from build123d import *

# Parameters (mm, degrees)
F0_R     = 140
F0_R_2   = 12.7
F0_R_3   = 87.5
F1_DEPTH = 15


with BuildPart() as f1:
    # F0 (on Front) → F1 (new body)
    with BuildSketch(Plane.XZ):
        Circle(F0_R)
        with Locations((-82.943625, -82.943625)):
            Circle(F0_R_2, mode=Mode.SUBTRACT)
        with Locations((0, -117.3)):
            Circle(F0_R_2, mode=Mode.SUBTRACT)
        with Locations((82.943625, -82.943625)):
            Circle(F0_R_2, mode=Mode.SUBTRACT)
        with Locations((-117.3, 0)):
            Circle(F0_R_2, mode=Mode.SUBTRACT)
        with Locations((-82.943625, 82.943625)):
            Circle(F0_R_2, mode=Mode.SUBTRACT)
        Circle(F0_R_3, mode=Mode.SUBTRACT)
        with Locations((117.3, 0)):
            Circle(F0_R_2, mode=Mode.SUBTRACT)
        with Locations((0, 117.3)):
            Circle(F0_R_2, mode=Mode.SUBTRACT)
        with Locations((82.943625, 82.943625)):
            Circle(F0_R_2, mode=Mode.SUBTRACT)
    extrude(amount=F1_DEPTH)


solid = f1.part
Part model, mm, in its own coordinate system. Give positions to 0.01 mm unless a question says otherwise; leave off trailing zeros. Loops run counter-clockwise (first coordinate to the right, second up) from the corner with the lowest first, then second, coordinate; pieces in that order, holes last.
(1) Band-saw the part on D-D (y = -10). Count the separate pieces of the cut face and the enclosed holes in it, and give its area (3 significant figures).
Return value:
separate pieces: 1
enclosed holes: 9
area: 33,500 mm2
(2) Drill centre lines: line 1 along Z through (x, y) = (0, -9); line 2 along Z through (x, y) = (79, -0.75); line 3 along Z through (x, y) = (-94.5, -8.5). Where is each one in solid material? Low to high.
Return value:
line 1: z = -140 to -130, -104.6 to -87.5, 87.5 to 104.6, 130 to 140
line 2: z = -115.58 to -95.02, -70.87 to -37.62, 37.62 to 70.87, 95.02 to 115.58
line 3: z = -103.29 to -88.21, -77.68 to 77.68, 88.21 to 103.29
(3) Band-saw the part on A-A (z = 0). Write the cut outline in (x, y).
Return value:
outline: (-140, -15) - (-130, -15) - (-130, 0) - (-140, 0) - close; (-104.6, -15) - (-87.5, -15) - (-87.5, 0) - (-104.6, 0) - close; (87.5, -15) - (104.6, -15) - (104.6, 0) - (87.5, 0) - close; (130, -15) - (140, -15) - (140, 0) - (130, 0) - close
(4) Pull direction Z, two halves, no side cores. Call faces 1 (the flat face through (60, -15, 64)), 2 (the cylindrical face through (-111.1, -7.4, -85.19)), 3 (the cylindrical face through (-1.653, -7.395, -104.708)), 4 (the cylindrical face through (-85.697, -7.395, 70.546)): pulls with the +Z half, pulls with the -Z half, needs draft (parallel to the pull), parting line crosses it, or undercut.
Return value:
face 1: needs draft
face 2: parting line crosses it
face 3: undercut
face 4: undercut
(5) Band-saw the part on B-B (x = -7). Write the cut outline in (y, z).
Return value:
outline: (-15, -139.82) - (0, -139.82) - (0, -127.9) - (-15, -127.9) - close; (-15, -106.7) - (0, -106.7) - (0, -87.22) - (-15, -87.22) - close; (-15, 87.22) - (0, 87.22) - (0, 106.7) - (-15, 106.7) - close; (-15, 127.9) - (0, 127.9) - (0, 139.82) - (-15, 139.82) - close
(6) Band-saw the part on C-C (x = 38). Write the cut outline in (y, z).
Return value:
outline: (-15, -134.74) - (0, -134.74) - (0, -78.82) - (-15, -78.82) - close; (-15, 78.82) - (0, 78.82) - (0, 134.74) - (-15, 134.74) - close
(7) Pin check, flat tips, straight feed: pin 1 (3 mm diameter, centred on x = 60.5, y = -9.5, fed in from -Z); pin 2 (15 mm diameter, centred on x = -82.94, z = -82.94, fed in from -Y) (3 decimals); pin 3 (6 mm diameter, centred on y = -5.5, z = 92, fed in from +X). Stop position of each tip, or through.
Return value:
pin 1: stops at z = -126.96
pin 2: passes through
pin 3: stops at x = 108.07
